Read the model definition and answer for the solid it produces. Units are mm, in the model's axes. Give positions to 0.01 mm unless a question says otherwise; leave off trailing zeros. Order: outer loops, then holes, each group sorted by start corner. A loop starts at its lowest first (then second) coordinate and runs counter-clockwise, first axis right, second up.
```python
from build123d import *

# Parameters (mm, degrees)
SKETCH2_W           = 80
SKETCH2_H           = 30
SKETCH2_R           = 10
SKETCH2_R_2         = 2.641043536
BOSS_EXTRUDE1_DEPTH = 5
FILLET2_R           = 5


with BuildPart() as part:
    # Sketch2 → Boss-Extrude1 (new body)
    with BuildSketch(Plane.XY):
        with Locations((0.618817107, -21.917958992)):
            Rectangle(SKETCH2_W, SKETCH2_H)
        with Locations((-19.381182893, -21.917958992)):
            Circle(SKETCH2_R, mode=Mode.SUBTRACT)
        with Locations((20.618817107, -21.917958992)):
            Circle(SKETCH2_R, mode=Mode.SUBTRACT)
        with Locations((0.618817107, -21.917958992)):
            Circle(SKETCH2_R_2, mode=Mode.SUBTRACT)
    extrude(amount=BOSS_EXTRUDE1_DEPTH)

    # Fillet2
    fillet2_edges = [part.edges().sort_by_distance(p)[0] for p in [
        (-39.381182893, -6.917958992, 2.5),
        (40.618817107, -6.917958992, 2.5),
    ]]
    fillet(fillet2_edges, radius=FILLET2_R)


solid = part.part
```
1) The part is cut by section A-A on y = -21. Determine the outline of the cut face in (x, z).
Final values:
outline: (-39.38, 0) - (-29.34, 0) - (-29.34, 5) - (-39.38, 5) - close; (-9.42, 0) - (-1.86, 0) - (-1.86, 5) - (-9.42, 5) - close; (3.1, 0) - (10.66, 0) - (10.66, 5) - (3.1, 5) - close; (30.58, 0) - (40.62, 0) - (40.62, 5) - (30.58, 5) - close
2) The part is cut by section C-C on x = 23. Determine the outline of the cut face in (y, z).
Final values:
outline: (-36.92, 0) - (-31.63, 0) - (-31.63, 5) - (-36.92, 5) - close; (-12.21, 0) - (-6.92, 0) - (-6.92, 5) - (-12.21, 5) - close
3) Consider L1, parallel to X at y = -19.75, z = 2.5; L2, parallel to X at y = -15.75, z = 2.1; L3, parallel to X at y = -17, z = 3.15. Determine where each line is inside the solid, lowest interval first.
Final values:
L1: x = -39.38 to -29.14, -9.62 to -0.89, 2.13 to 10.86, 30.38 to 40.62
L2: x = -39.38 to -27.25, -11.51 to 12.75, 28.49 to 40.62
L3: x = -39.38 to -28.09, -10.67 to 11.91, 29.33 to 40.62
4) For a pull along Y with two mould halves and no side action, classify faces 1 (the face through (39.115, -8.344, 2.535)), 2 (the face through (18.45, -31.68, 2.46)), 3 (the face through (40.619, -25, 2)) as released by +Y, released by -Y, zero draft, split by the parting line, or undercut.
Final values:
face 1: released by +Y
face 2: undercut
face 3: zero draft
5) Given pin 1 (12 mm diameter, centred on x = 20.62, y = -21.92, fed in from -Z), flat-ended and moving along its own axis, determine where the tip first touches the part or whether it passes through.
Final values:
pin 1: passes through
6) The part is cut by section B-B on y = -26.75. Determine the outline of the cut face in (x, z), and give its area (3 significant figures).
Final values:
outline: (-39.38, 0) - (-28.14, 0) - (-28.14, 5) - (-39.38, 5) - close; (-10.63, 0) - (11.86, 0) - (11.86, 5) - (-10.63, 5) - close; (29.37, 0) - (40.62, 0) - (40.62, 5) - (29.37, 5) - close
area: 225 mm2
7) The part is cut by section D-D on z = 1.6. Determine the outline of the cut face in (x, y), and give its area (3 significant figures).
Final values:
outline: (-39.38, -36.92) - (40.62, -36.92) - (40.62, -11.92) arc R5 ccw to (35.62, -6.92) - (-34.38, -6.92) arc R5 ccw to (-39.38, -11.92) - close; hole circle Ø20 at (-19.38, -21.92); hole circle Ø5.28 at (0.62, -21.92); hole circle Ø20 at (20.62, -21.92)
area: 1,740 mm2
